Design review of the part built by this model. Coordinates are the model's own, in mm. A direction names the side the tool comes from. Give positions to 0.01 mm unless a question says otherwise; leave off trailing zeros. Write each loop counter-clockwise with the first axis right and the second up, starting at its lowest first coordinate (ties: lowest second). Pieces come first, ordered by that corner, then holes. Notation, with made-up numbers: (-35, 11) -> (-22, 11) arc R10 cw to (-22, 23) -> close; hole circle Ø2 at (53.5, 44). An arc over 180 degrees is marked (long way). Answer as a JSON object with one key per item and string values.
```python
from build123d import *

# Parameters (mm, degrees)
SKETCH1_R            = 4
BOSS_EXTRUDE1_DEPTH  = 7
SKETCH2_R            = 6
BOSS_EXTRUDE2_DEPTH  = 0.5
BOSS_EXTRUDE3_START  = 0.5
SKETCH3_R            = 6
BOSS_EXTRUDE3_DEPTH  = 0.5
M3_CLEARANCE_HOLE1_D = 3.2
FILLET1_R            = 0.5


with BuildPart() as part:
    # Sketch1 → Boss-Extrude1 (new body)
    with BuildSketch(Plane(origin=(0, 0, 0), x_dir=(1, 0, 0), z_dir=(0, 1, 0))):
        with Locations(Location((0, 0, 0), (0, 0, 270))):
            Circle(SKETCH1_R)
    extrude(amount=BOSS_EXTRUDE1_DEPTH)

    # Sketch2 → Boss-Extrude2 (add)
    with BuildSketch(Plane(origin=(0, 7, 0), x_dir=(1, 0, 0), z_dir=(0, 1, 0))):
        with Locations(Location((0, 0, 0), (0, 0, 270))):
            Circle(SKETCH2_R)
    extrude(amount=BOSS_EXTRUDE2_DEPTH)

    # Sketch3 → Boss-Extrude3 (add)
    with BuildSketch(Plane.XZ.offset(BOSS_EXTRUDE3_START)):
        with Locations(Location((0, 0, 0), (0, 0, 90))):
            Circle(SKETCH3_R)
    extrude(amount=-BOSS_EXTRUDE3_DEPTH)

    # M3 Clearance Hole1 (through all)
    with Locations(Plane(origin=(0, -0.5, 0), x_dir=(-1, 0, 0), z_dir=(0, -1, 0))):
        with Locations((0, 0)):
            Hole(M3_CLEARANCE_HOLE1_D / 2)

    # Fillet1
    fillet1_edges = [part.edges().sort_by_distance(p)[0] for p in [
        (0, 7, -4),
        (0, 0, -4),
    ]]
    fillet(fillet1_edges, radius=FILLET1_R)


solid = part.part
```
(1) For faces 1 (the cylindrical face through (1.802, 7.246, 5.723)), 2 (the cylindrical face through (-3.905, 3.458, -0.867)), list the 3-axis set-ups (+Z, -Z, +X, -X, +Y, -Y) from which the entire face can be reached by the end or side of a thin tool; tool diameter is ignored.
Here are the results:
{"face 1": "+Y, -Y", "face 2": "none"}
(2) We need section B-B, the plane z = 0. State the section outline as (x, y) points.
Here are the results:
{"outline": "(-6, -0.5) -> (-1.6, -0.5) -> (-1.6, 7.5) -> (-6, 7.5) -> (-6, 7) -> (-4.5, 7) arc R0.5 cw to (-4, 6.5) -> (-4, 0.5) arc R0.5 cw to (-4.5, 0) -> (-6, 0) -> close; (1.6, -0.5) -> (6, -0.5) -> (6, 0) -> (4.5, 0) arc R0.5 cw to (4, 0.5) -> (4, 6.5) arc R0.5 cw to (4.5, 7) -> (6, 7) -> (6, 7.5) -> (1.6, 7.5) -> close"}
(3) For line 1 along Y through (x, z) = (3, 5); line 2 along X through (y, z) = (4.25, 1.25); line 3 along X through (y, z) = (3.5, -2.25), list the stretches that pass through material, from the lowest coordinate up.
Here are the results:
{"line 1": "y = -0.5 to 0, 7 to 7.5", "line 2": "x = -3.8 to -1, 1 to 3.8", "line 3": "x = -3.31 to 3.31"}
(4) We need section D-D, the plane x = 5. State the section outline as (y, z) points.
Here are the results:
{"outline": "(-0.5, -3.32) -> (0, -3.32) -> (0, 3.32) -> (-0.5, 3.32) -> close; (7, -3.32) -> (7.5, -3.32) -> (7.5, 3.32) -> (7, 3.32) -> close"}
(5) Clearance check with a flat-ended pin moving along its axis: pin 1 (1.5 mm diameter, centred on y = 6, z = 0.5, fed in from +X). State where the tip first meets the part, or that it passes through.
Here are the results:
{"pin 1": "stops at x = 4.04"}
(6) We need section A-A, the plane x = 0. State the section outline as (y, z) points, then the cut area to 3 significant figures.
Here are the results:
{"outline": "(-0.5, -6) -> (0, -6) -> (0, -4.5) arc R0.5 cw to (0.5, -4) -> (6.5, -4) arc R0.5 cw to (7, -4.5) -> (7, -6) -> (7.5, -6) -> (7.5, -1.6) -> (-0.5, -1.6) -> close; (-0.5, 1.6) -> (7.5, 1.6) -> (7.5, 6) -> (7, 6) -> (7, 4.5) arc R0.5 cw to (6.5, 4) -> (0.5, 4) arc R0.5 cw to (0, 4.5) -> (0, 6) -> (-0.5, 6) -> close", "area": "42.6 mm²"}
(7) The part is to be moulded in two halves that separate along Y. For faces 3 (the flat face through (1.25, -0.5, 1.25)), 4 (the flat face through (4.5, 7, -1.4)), 5 (the cylindrical face through (-1.802, -0.254, 5.723)), say which applies: +Y half, -Y half, draft (parallel to the pull), parting line (faces both ways), or undercut.
Here are the results:
{"face 3": "-Y half", "face 4": "undercut", "face 5": "draft"}
(8) We need section C-C, the plane y = 2.25. State the section outline as (x, z) points.
Here are the results:
{"outline": "circle Ø8 at (0, 0); hole circle Ø3.2 at (0, 0)"}
